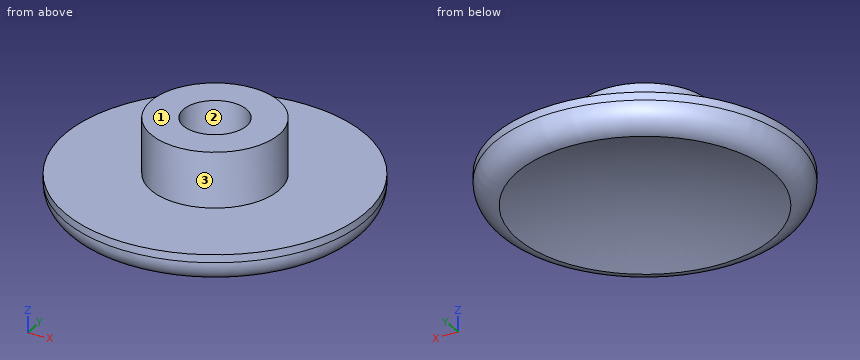
```python
from build123d import *

# Parameters (mm, degrees)
F0_R     = 9.5
F0_R_2   = 4.05
F0_R_3   = 2
F1_DEPTH = 2
F2_R     = 4.05
F2_R_2   = 2
F3_DEPTH = 5.5
F4_R     = 1.5


# Not quite as in the source:
# - a feature names something its author has since deleted; it is built from what else it names


with BuildPart() as f1:
    # F0 (on Top) → F1 (new body)
    with BuildSketch(Plane.XY):
        Circle(F0_R)
        Circle(F0_R_2, mode=Mode.SUBTRACT)
        Circle(F0_R_2)
        Circle(F0_R_3, mode=Mode.SUBTRACT)
        Circle(F0_R_3)
    extrude(amount=F1_DEPTH)

    # F2 (on Top) → F3 (join)
    with BuildSketch(Plane.XY):
        Circle(F2_R)
        Circle(F2_R_2, mode=Mode.SUBTRACT)
    extrude(amount=F3_DEPTH)

    # F4
    f4_edges = [f1.edges().sort_by_distance(p)[0] for p in [
        (-9.5, 0, 0),
    ]]
    fillet(f4_edges, radius=F4_R)

    # F5 (on Front) → F6 (revolve, cut)
    with BuildSketch(Plane.XZ):
        with BuildLine():
            ThreePointArc((0, 0), (23.1570723538, -9.489364109), (32.9962119038, -32.5))
            ThreePointArc((32.9962119038, -32.5), (23.510635891, -8.8429276462), (0, 1))
            Line((0, 1), (0, 0))
        make_face()
    revolve(axis=Axis((0, 0, -31.5146126637), (0, 0, -1)), mode=Mode.SUBTRACT)


solid = f1.part
```
Check sheet for the modelled part. Datum: model origin and axes. Units: mm. Face numbers are marked on the shaded views. Round coordinates to 2 decimals unless told otherwise and drop trailing zeros. Loops run counter-clockwise (first coordinate to the right, second up) from the corner with the lowest first, then second, coordinate; pieces in that order, holes last. Notation, with made-up numbers: (-32, 17) -> (-21, 17) arc R33 ccw to (-21, 54) -> close; hole circle Ø3 at (31.25, -11.75). An arc over 180 degrees is marked (long way). Write item = value, one per line. Start each with the question number.
1) Sectioned sample at A-A, the plane x = 0. Record the cut outline in (y, z).
2) Gauge pin test, flat ends, axial feed: pin 1 Ø1.5 at (x, z) = (-6, 2.5) entering from -Y; pin 2 Ø2 at (y, z) = (4, 4.5) entering from +X; pin 3 Ø3 at (x, y) = (0, 0) entering from +Z. Record the tip position at first contact, or that the pin passes through.
3) Thickness scan on probe 1 along X at (y, z) = (0, 2.75); probe 2 along Y at (x, z) = (1.75, 3.8). Record the ranges inside material, lowest first.
4) Release check for a two-part mould opening along Y. For the marked faces 1, 2 and 3 record: released by +Y, released by -Y, zero draft, split by the parting line, or undercut.
5) Sectioned sample at C-C, the plane z = 3.15. Record the cut outline in (x, y).
Results are:
q1.outline = (-9.5, 1.5) arc R1.5 ccw to (-8.06, 0) arc R33 cw to (8.06, 0) arc R1.5 ccw to (9.5, 1.5) -> (9.5, 2) -> (4.05, 2) -> (4.05, 5.5) -> (2, 5.5) -> (2, 2) -> (-2, 2) -> (-2, 5.5) -> (-4.05, 5.5) -> (-4.05, 2) -> (-9.5, 2) -> close
q2.pin_1 = -7.79
q2.pin_2 = 2.72
q2.pin_3 = 2
q3.probe_1 = -4.05 to -2, 2 to 4.05
q3.probe_2 = -3.65 to -0.97, 0.97 to 3.65
q4.face_1 = zero draft
q4.face_2 = undercut
q4.face_3 = split by the parting line
q5.outline = circle Ø8.1 at (0, 0); hole circle Ø4 at (0, 0)
